Check sheet for the modelled part. Datum: model origin and axes. Units: mm. A direction names the side the tool comes from. Round coordinates to 2 decimals unless told otherwise and drop trailing zeros. Write each loop counter-clockwise with the first axis right and the second up, starting at its lowest first coordinate (ties: lowest second). Pieces come first, ordered by that corner, then holes. Notation, with made-up numbers: (-31, 53.25) - (20, 53.25) arc R9 cw to (20, 67.25) - close; hole circle Ø8 at (-33, 78.25). An arc over 180 degrees is marked (long way). Answer as a JSON object with one key per item and string values. Group by question number.
Item 1: Sectioned sample at B-B on y = 6. Record the boundary of the cut face in (x, z).
Item 2: Sectioned sample at C-C on x = 5. Record the boundary of the cut face in (y, z).
Item 3: Sectioned sample at D-D on y = -14. Record the boundary of the cut face in (x, z), plus the area to 3 significant figures.
Item 4: Thickness scan on line 1 (X direction, y = -2.5, z = 0.2); line 2 (Y direction, x = -3.5, z = 0.4); line 3 (X direction, y = 17, z = 0.1). Record the ranges inside material, lowest first.
Item 5: Sectioned sample at A-A on z = 0.3. Record the boundary of the cut face in (x, y) (1 decimal), plus the area to 3 significant figures.
Item 6: Release check for a two-part mould opening along X. For faces 1 (the flat face through (-5, 0, 0)), 2 (the cylindrical face through (-4.336, -19.524, 0.246)), 3 (the cylindrical face through (1.49, 0.47, 0.25)) record: pulls with the +X half, pulls with the -X half, needs draft (parallel to the pull), parting line crosses it, or undercut.
Item 7: Gauge pin test, flat ends, axial feed: P1, Ø8, axis at x = -9, y = -3, coming from the -Z side; P2, Ø3, axis at x = 0, y = 0, coming from the -Z side. Record the tip position at first contact, or that the pin passes through.
Item 8: Set-up check for faces 4 (the flat face through (-5, 0, 0.5)), 5 (the cylindrical face through (-3.32, 5.66, 0.25)): record each of +Z, -Z, +X, -X, +Y, -Y from which the full face is reachable in a straight line by a thin tool's end or side.
```python
from build123d import *

# Parameters (mm, degrees)
F0_R     = 20
F0_R_2   = 1.5625
F1_DEPTH = 0.5


with BuildPart() as f1:
    # F0 (on Top) → F1 (new body)
    with BuildSketch(Plane.XY):
        Circle(F0_R)
        with BuildLine():
            ThreePointArc((-5.683292, -3.28125), (-5.111377, -1.146835), (-2.976962, -1.71875))
            ThreePointArc((-2.976962, -1.71875), (-1.71875, -2.976962), (0, -3.4375))
            ThreePointArc((0, -3.4375), (1.5625, -5), (0, -6.5625))
            ThreePointArc((0, -6.5625), (-3.28125, -5.683292), (-5.683292, -3.28125))
        make_face(mode=Mode.SUBTRACT)
        with BuildLine():
            ThreePointArc((0, 6.5625), (1.5625, 5), (0, 3.4375))
            ThreePointArc((0, 3.4375), (-1.71875, 2.976962), (-2.976962, 1.71875))
            ThreePointArc((-2.976962, 1.71875), (-5.111377, 1.146835), (-5.683292, 3.28125))
            ThreePointArc((-5.683292, 3.28125), (-3.28125, 5.683292), (0, 6.5625))
        make_face(mode=Mode.SUBTRACT)
        Circle(F0_R_2, mode=Mode.SUBTRACT)
        with BuildLine():
            ThreePointArc((5.683292, -3.28125), (3.548877, -3.853165), (2.976962, -1.71875))
            ThreePointArc((2.976962, -1.71875), (3.4375, 0), (2.976962, 1.71875))
            ThreePointArc((2.976962, 1.71875), (3.548877, 3.853165), (5.683292, 3.28125))
            ThreePointArc((5.683292, 3.28125), (6.5625, 0), (5.683292, -3.28125))
        make_face(mode=Mode.SUBTRACT)
    extrude(amount=F1_DEPTH)


solid = f1.part
```
Completed:
{
 "1": {"outline": "(-19.08, 0) - (-2.66, 0) - (-2.66, 0.5) - (-19.08, 0.5) - close; (1.2, 0) - (19.08, 0) - (19.08, 0.5) - (1.2, 0.5) - close"},
 "2": {"outline": "(-19.36, 0) - (-3.91, 0) - (-3.91, 0.5) - (-19.36, 0.5) - close; (3.91, 0) - (19.36, 0) - (19.36, 0.5) - (3.91, 0.5) - close"},
 "3": {"outline": "(-14.28, 0) - (14.28, 0) - (14.28, 0.5) - (-14.28, 0.5) - close", "area": "14.3 mm²"},
 "4": {"line 1": "-19.84 to -5.89, -2.36 to 2.77, 6.07 to 19.84", "line 2": "-19.69 to -5.55, -1.18 to 1.18, 5.55 to 19.69", "line 3": "-10.54 to 10.54"},
 "5": {"outline": "circle Ø40 at (0, 0); hole (-5.7, -3.3) arc R6.6 ccw to (0, -6.6) arc R1.6 ccw to (0, -3.4) arc R3.4 cw to (-3, -1.7) arc R1.6 ccw to start; hole (-5.7, 3.3) arc R1.6 ccw to (-3, 1.7) arc R3.4 cw to (0, 3.4) arc R1.6 ccw to (0, 6.6) arc R6.6 ccw to start; hole circle Ø3.1 at (0, 0); hole (3, -1.7) arc R1.6 ccw to (5.7, -3.3) arc R6.6 ccw to (5.7, 3.3) arc R1.6 ccw to (3, 1.7) arc R3.4 cw to start", "area": "1,180 mm²"},
 "6": {"face 1": "needs draft", "face 2": "parting line crosses it", "face 3": "undercut"},
 "7": {"P1": "z = 0", "P2": "through"},
 "8": {"face 4": "+Z, +X, -X, +Y, -Y", "face 5": "+Z, -Z"}
}
